Autodesk Inventor part; units mm, degrees
ref_plane "YZ Plane" through (0, 0, 0) normal (1, 0, 0) x (0, 1, 0)
ref_plane "XZ Plane" through (0, 0, 0) normal (0, 1, 0) x (-1, 0, 0)
ref_plane "XY Plane" through (0, 0, 0) normal (0, 0, 1) x (1, 0, 0)
sketch "Skizze3" plane through (0, 0, 0) normal (0, 1, 0) x (-1, 0, 0)
  line L0 (5, -5) -> (5, -25)
  line L1 (5, -25) -> (0, -25)
  line L2 (0, -25) -> (0, 0)
  line L3 (0, 0) -> (5, -5)
  dimension "d7" = 5
  dimension "d11" = 25
  dimension "d12" = 20
extrude "Extrusion3" add sketch "Skizze3" along normal blind 8
sketch "Skizze4" plane through (0, 0, 0) normal (1, 0, 0) x (0, 0, -1)
  line L0 (-0.7299, 4) -> (5.994, 4) construction
  line L1 (0, 0) -> (0, 8)
  point P0 (17, 4)
  point P1 (0, 4)
  dimension "d10" = 17
hole "Bohrung1" at (0, 4, -17) direction (-1, 0, 0) diameter 3.4 end through all counterbore diameter 6 counterbore depth 3.4
chamfer "Fase1" distance 2 angle 45 1 edges at (-5, 4, -25)
mirror "Spiegeln1" about plane through (-5, 0, -5) normal (-0.7071, 0, 0.7071) of "Extrusion3", "Bohrung1", "Fase1"
sketch "Skizze5" plane through (0, 0, -25) normal (1, 0, 0) x (0, 0, -1)
  line L0 (-25, 8) -> (0, 8)
  line L1 (-25, 0) -> (-25, 8)
  line L2 (-25, 8) -> (0, 8)
  line L3 (0, 8) -> (0, 10)
  line L4 (0, 10) -> (-25, 10)
  line L5 (-25, 10) -> (-25, 8)
  dimension "d23" = 2
extrude "Extrusion4" add sketch "Skizze5" against normal blind 25
sketch "Skizze6" plane through (0, 10, 0) normal (0, 1, 0) x (1, 0, 0)
  line L0 (-3, 25) -> (-25, 25)
  line L1 (-3, 25) -> (-25, 3)
  line L2 (0, 25) -> (-25, 25)
  line L3 (-25, 0) -> (-25, 25)
  point P0 (0, 0)
extrude "Extrusion5" cut sketch "Skizze6" against normal blind 10
equation "\"d12\" = d11 - d7"
properties part number "BT406_trajan20_21" material "Kunststoff, undurchsichtig Schwarz"
Part model, mm, in its own coordinate system. A direction names the side the tool comes from. Give positions to 0.01 mm unless a question says otherwise; leave off trailing zeros. Order: outer loops, then holes, each group sorted by start corner. A loop starts at its lowest first (then second) coordinate and runs counter-clockwise, first axis right, second up. Notation, with made-up numbers: M 57.5,24 L 75.5,24 A6 cw 75.5,29 Z; hole C 78.5,58.25 d7. An arc over 180 degrees is marked long. Use a Markdown table: item, result. Add a question column.
(1) Saw through at B-B, the plane x = -17. Give the cut face in (y, z), and give its area (3 significant figures).
(2) Drop flat-ended pins along their axis: P1, Ø1.5, axis at y = 4, z = -7, coming from the -X side; P2, Ø4.5, axis at x = -17, y = 4, coming from the -Z side; P3, Ø3.5, axis at y = 4, z = -17, coming from the +X side; P4, Ø3, axis at y = 7, z = -11.5, coming from the +X side. Give the stop position or say it passes through.
(3) 3-axis set-ups, long thin cutter, end or side, ignore diameter. For faces 4 (the face through (-14.6, 2.2, -1.7)), 5 (the face through (-3.4, 4, -19)), 6 (the face through (-5, 4, -14)): which of +Z, -Z, +X, -X, +Y, -Y reach the whole face in a straight line?
(4) Probe line 1 along Y through (x, z) = (-17, -1.7); line 2 along Y through (x, z) = (-4.2, -17); line 3 along X through (y, z) = (4, -2.2). List the from-to ranges inside material, lowest first. Write a range as [from, to].
(5) Saw through at A-A, the plane z = -17. Give the cut face in (x, y), and give its area (3 significant figures).
(6) Saw through at D-D, the plane y = 8.5. Give the cut face in (x, z), and give its area (3 significant figures).
(7) Mould opens along X. For faces 1 (the face through (0, 5, -12)), 2 (the face through (-7, 0, -4)), 3 (the face through (-18.57, 3.35, -4.21)) say: +X half, -X half, draft (parallel to the pull), parting line (faces both ways), or undercut.
(8) Saw through at C-C, the plane y = 4. Give the cut face in (x, z).
Answer key:
| question | item | result |
|---|---|---|
| 1 | outline | M 0,-5 L 2.3,-5 L 2.3,-3.4 L 1,-3.4 L 1,0 L 0,0 Z; M 5.7,-5 L 8,-5 L 8,-11 L 10,-11 L 10,0 L 7,0 L 7,-3.4 L 5.7,-3.4 Z |
| 1 | area | 36.2 mm^2 |
| 2 | P1 | x = -5 |
| 2 | P2 | z = -5 |
| 2 | P3 | x = -3.4 |
| 2 | P4 | x = 0 |
| 3 | face 4 | +Z |
| 3 | face 5 | +X |
| 3 | face 6 | -Z, -X, -Y |
| 4 | line 1 | [0, 1], [7, 10] |
| 4 | line 2 | [0, 2.3], [5.7, 10] |
| 4 | line 3 | [-25, -20], [-14, 0] |
| 5 | outline | M -11,8 L -5,8 L -5,5.7 L -3.4,5.7 L -3.4,7 L 0,7 L 0,10 L -11,10 Z; M -5,0 L 0,0 L 0,1 L -3.4,1 L -3.4,2.3 L -5,2.3 Z |
| 5 | area | 36.2 mm^2 |
| 6 | outline | M -25,-3 L -3,-25 L 0,-25 L 0,0 L -25,0 Z |
| 6 | area | 383 mm^2 |
| 7 | face 1 | +X half |
| 7 | face 2 | draft |
| 7 | face 3 | undercut |
| 8 | outline | M -25,-3 L -23,-5 L -18.7,-5 L -18.7,-3.4 L -20,-3.4 L -20,0 L -25,0 Z; M -15.3,-5 L -5,-5 L -5,-15.3 L -3.4,-15.3 L -3.4,-14 L 0,-14 L 0,0 L -14,0 L -14,-3.4 L -15.3,-3.4 Z; M -5,-23 L -3,-25 L 0,-25 L 0,-20 L -3.4,-20 L -3.4,-18.7 L -5,-18.7 Z |
